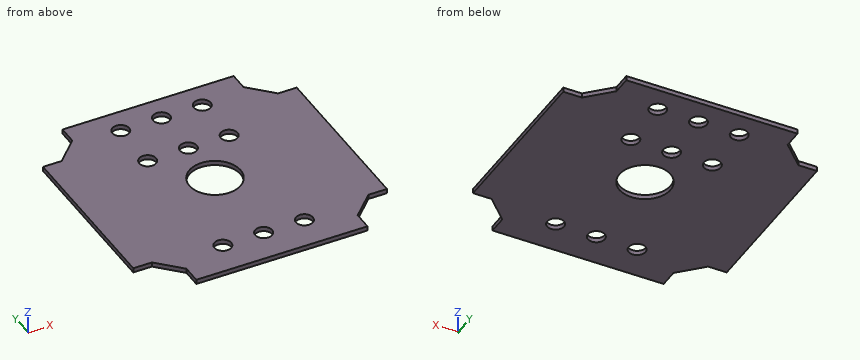
Autodesk Inventor part; units mm, degrees
ref_plane "Work Plane1" through (-29.1, -14.5, 2.4) normal (0, 0, -1) x (0, 1, 0)
ref_plane "Work Plane2" through (-15, -33.1, 1.9) normal (0, 0, -1) x (0, 1, 0)
ref_plane "Work Plane3" through (14, -23.1, 0.9) normal (0, 0, -1) x (0, 1, 0)
ref_plane "Work Plane1" through (-29.1, -14.5, 2.4) normal (0, 0, -1) x (0, 1, 0)
ref_plane "Work Plane2" through (-15, -33.1, 1.9) normal (0, 0, -1) x (0, 1, 0)
ref_plane "Work Plane3" through (14, -23.1, 0.9) normal (0, 0, -1) x (0, 1, 0)
sketch "Sketch1" plane through (0, 0, 0) normal (0, 0, 1) x (1, 0, 0)
  line L0 (-34.86, 0) -> (34.86, 0) construction
  line L1 (0, -34.86) -> (0, 34.86) construction
  line L2 (0, 0) -> (11.1575, 11.1575) construction
  line L3 (0, 0) -> (15.7791, 0) construction
  line L4 (0, 24.9) -> (16.8009, 24.9)
  line L5 (16.8009, 24.9) -> (16.8009, 21.2415)
  line L6 (16.8009, 21.2415) -> (19.0212, 19.0212)
  line L7 (24.9, 0) -> (24.9, 16.8009)
  line L8 (24.9, 16.8009) -> (21.2415, 16.8009)
  line L9 (21.2415, 16.8009) -> (19.0212, 19.0212)
  line L10 (0, -24.9) -> (16.8009, -24.9)
  line L11 (16.8009, -24.9) -> (16.8009, -21.2415)
  line L12 (16.8009, -21.2415) -> (19.0212, -19.0212)
  line L13 (24.9, 0) -> (24.9, -16.8009)
  line L14 (24.9, -16.8009) -> (21.2415, -16.8009)
  line L15 (21.2415, -16.8009) -> (19.0212, -19.0212)
  line L16 (0, 24.9) -> (-16.8009, 24.9)
  line L17 (-16.8009, 24.9) -> (-16.8009, 21.2415)
  line L18 (-16.8009, 21.2415) -> (-19.0212, 19.0212)
  line L19 (-24.9, 16.8009) -> (-21.2415, 16.8009)
  line L20 (-21.2415, 16.8009) -> (-19.0212, 19.0212)
  line L21 (0, -24.9) -> (-16.8009, -24.9)
  line L22 (-16.8009, -24.9) -> (-16.8009, -21.2415)
  line L23 (-16.8009, -21.2415) -> (-19.0212, -19.0212)
  line L24 (-21.2415, -16.8009) -> (-19.0212, -19.0212)
  line L25 (-24.9, -16.8009) -> (-21.2415, -16.8009)
  line L26 (-24.9, 0) -> (-24.9, -16.8009)
  line L27 (-24.9, 0) -> (-24.9, 16.8009)
  circle A0 centre (0, 0) radius 5
  dimension "d0" = 45
  dimension "d2" = 24.9
  dimension "d3" = 3.14
  dimension "d4" = 26.9
  dimension "d5" = 10
extrude "Extrusion1" add sketch "Sketch1" along normal up to surface (0.9 mm away)
sketch "Sketch5" plane through (0, 0, 0) normal (0, 0, -1) x (-1, 0, 0)
  circle A0 centre (-8, -18.1) radius 1.4 construction
  circle A1 centre (0, -18.1) radius 1.4 construction
  circle A2 centre (8, -18.1) radius 1.4 construction
  circle A3 centre (-12, -18.1) radius 1.4 construction
  circle A4 centre (0, 9.9) radius 1.4 construction
  circle A5 centre (-8, 9.9) radius 1.4 construction
  circle A6 centre (8, 9.9) radius 1.4 construction
  circle A7 centre (8, 19.9) radius 1.4 construction
  circle A8 centre (0, 19.9) radius 1.4 construction
  circle A9 centre (-8, 19.9) radius 1.4 construction
  point P0 (-9.7, 10)
  point P1 (-9.7, -10)
  point P2 (13.8, 0)
  point P3 (-0.2419, -17.9861)
hole "Hole1" at (8, 19.9, 0) at (0, 19.9, 0) at (-8, 19.9, 0) at (0, -18.1, 0) at (-8, -18.1, 0) at (8, 9.9, 0) at (0, 9.9, 0) at (-8, 9.9, 0) at (8, -18.1, 0) direction (0, 0, 1) diameter 3.3 depth 12 tip angle 118
properties part number "20_Cube_insert_Sample_holder"
Check sheet for the modelled part. Datum: model origin and axes. Units: mm. Round coordinates to 2 decimals unless told otherwise and drop trailing zeros. Loops run counter-clockwise (first coordinate to the right, second up) from the corner with the lowest first, then second, coordinate; pieces in that order, holes last. Notation, with made-up numbers: (7, -23) -> (57, -23) arc R32 ccw to (57, 4) -> close; hole circle Ø10 at (36.25, -16). An arc over 180 degrees is marked (long way). Put each result on its own line as item: value. Start each with the question number.
1. Section check C-C (z = 0.65). Give the number of separate pieces and of enclosed holes in the cut face, plus the area to 3 significant figures.
2. Section check B-B (x = -8). Enter the section's corners in (y, z), plus the area to 3 significant figures.
3. Gauge pin test, flat end, axial feed: pin 1 (4 mm diameter, centred on x = 8, y = 9.9, fed in from +Z). Record the tip position at first contact, or that the pin passes through.
4. Section check A-A (y = -3). Enter the section's corners in (x, z).
5. Scan lines: probe 1 along Y at (x, z) = (8, 0.5); probe 2 along X at (y, z) = (9.9, 0.6); probe 3 along Y at (x, z) = (0, 0.25). Record each from-to range of solid material in increasing order.
Findings:
1. separate pieces: 1
1. enclosed holes: 10
1. area: 2,100 mm^2
2. outline: (-24.9, 0) -> (-19.75, 0) -> (-19.75, 0.9) -> (-24.9, 0.9) -> close; (-16.45, 0) -> (8.25, 0) -> (8.25, 0.9) -> (-16.45, 0.9) -> close; (11.55, 0) -> (18.25, 0) -> (18.25, 0.9) -> (11.55, 0.9) -> close; (21.55, 0) -> (24.9, 0) -> (24.9, 0.9) -> (21.55, 0.9) -> close
2. area: 35.9 mm^2
3. pin 1: stops at z = 0.9
4. outline: (-24.9, 0) -> (-4, 0) -> (-4, 0.9) -> (-24.9, 0.9) -> close; (4, 0) -> (24.9, 0) -> (24.9, 0.9) -> (4, 0.9) -> close
5. probe 1: y = -24.9 to -19.75, -16.45 to 8.25, 11.55 to 18.25, 21.55 to 24.9
5. probe 2: x = -24.9 to -9.65, -6.35 to -1.65, 1.65 to 6.35, 9.65 to 24.9
5. probe 3: y = -24.9 to -19.75, -16.45 to -5, 5 to 8.25, 11.55 to 18.25, 21.55 to 24.9
